For this review, take the finished solid that the model builds, in its own axes (mm). Face numbers are marked on the shaded views. A direction names the side the tool comes from. Round coordinates to 2 decimals unless told otherwise and drop trailing zeros. Write each loop counter-clockwise with the first axis right and the second up, starting at its lowest first coordinate (ties: lowest second). Pieces come first, ordered by that corner, then holes. Notation, with made-up numbers: (9, -8.5) -> (58, -8.5) arc R24 cw to (58, 13.5) -> close; hole circle Ø4 at (-13, 9.25). An arc over 180 degrees is marked (long way). Answer as CSV lines item,"result". Start each with the question number.
Item 1: Mouldability with a two-part tool opening along Y and no side actions: class the marked faces 4, 5 and 6 as +Y half, -Y half, draft (parallel to the pull), parting line (faces both ways), or undercut.
Item 2: Machinability: for the marked faces 1, 2 and 3, which of the approach directions +Z, -Z, +X, -X, +Y, -Y give a long, thin tool a straight path to every point of the face, cutting with its end or side? Answer none if there is none.
Item 3: Wall thickness on probe 1 along Y at (x, z) = (-0.25, 2.5); probe 2 along Y at (x, z) = (-4, 9.75): over which ranges is each line inside the solid? List them lowest first. Write a range as from..to.
Item 4: Take a section at C-C on y = 0.25. Give the boundary of the cut face in (x, z).
Item 5: Take a section at D-D on x = -1.75. Give the boundary of the cut face in (y, z), then the cut area to 3 significant figures.
Item 6: Take a section at B-B on z = 8.5. Count the separate pieces of the cut face and the enclosed holes in it, then the cut area to 3 significant figures.
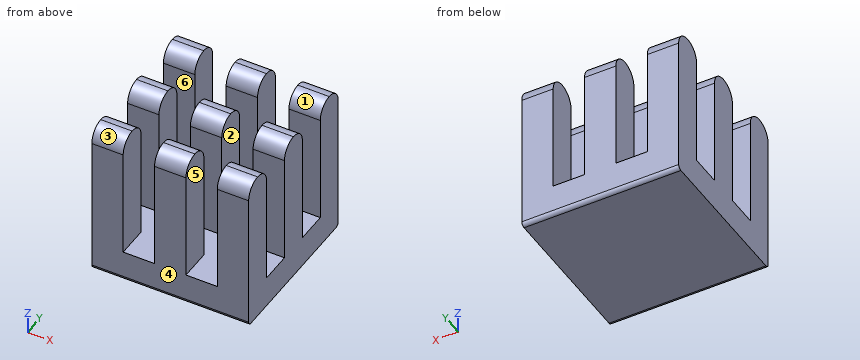
```python
from build123d import *

# Parameters (mm, degrees)
BOX_W                  = 10
BOX_H                  = 10
BOX_DEPTH              = 10
SKETCH_W               = 2
SKETCH_H               = 10
POCKET_DEPTH           = 10.001
LINEARPATTERN_COUNT    = 2
LINEARPATTERN_PITCH    = 4
SKETCH001_W            = 2
SKETCH001_H            = 10
POCKET001_DEPTH        = 10.001
LINEARPATTERN001_COUNT = 2
LINEARPATTERN001_PITCH = 4
FILLET_R               = 0.999
FILLET001_R            = 0.25


with BuildPart() as part:
    # Box → Box (new body)
    with BuildSketch(Plane(origin=(-5, -5, 0), x_dir=(1, 0, 0), z_dir=(0, 0, 1))):
        with Locations((5, 5)):
            Rectangle(BOX_W, BOX_H)
    extrude(amount=BOX_DEPTH)

    # Sketch → Pocket (cut, through all)
    with BuildSketch(Plane(origin=(-5, -5, 0), x_dir=(1, 0, 0), z_dir=(0, -1, 0))):
        with Locations((3, 7)):
            Rectangle(SKETCH_W, SKETCH_H)
    pocket = extrude(amount=-POCKET_DEPTH, mode=Mode.SUBTRACT)

    # LinearPattern: Pocket ×2
    with Locations(*[(i * LINEARPATTERN_PITCH, 0, 0) for i in range(1, LINEARPATTERN_COUNT)]):
        add(pocket, mode=Mode.SUBTRACT)

    # Sketch001 → Pocket001 (cut, through all)
    with BuildSketch(Plane(origin=(5, -5, 0), x_dir=(0, 1, 0), z_dir=(1, 0, 0))):
        with Locations((3, 7)):
            Rectangle(SKETCH001_W, SKETCH001_H)
    pocket001 = extrude(amount=-POCKET001_DEPTH, mode=Mode.SUBTRACT)

    # LinearPattern001: Pocket001 ×2
    with Locations(*[(0, i * LINEARPATTERN001_PITCH, 0) for i in range(1, LINEARPATTERN001_COUNT)]):
        add(pocket001, mode=Mode.SUBTRACT)

    # Fillet
    fillet_edges = [part.edges().sort_by_distance(p)[0] for p in [
        (-4, -5, 10),
        (-4, -3, 10),
        (0, -5, 10),
        (0, -3, 10),
        (4, -5, 10),
        (4, -3, 10),
        (4, -1, 10),
        (4, 1, 10),
        (0, 1, 10),
        (0, -1, 10),
        (-4, -1, 10),
        (-4, 1, 10),
        (-4, 3, 10),
        (-4, 5, 10),
        (0, 5, 10),
        (0, 3, 10),
        (4, 5, 10),
        (4, 3, 10),
    ]]
    fillet(fillet_edges, radius=FILLET_R)

    # Fillet001
    fillet001_edges = [part.edges().sort_by_distance(p)[0] for p in [
        (0, -5, 0),
        (0, 5, 0),
    ]]
    fillet(fillet001_edges, radius=FILLET001_R)


solid = part.part
```
Output values:
1,face 4,"-Y half"
1,face 5,"draft"
1,face 6,"undercut"
2,face 1,"+Z, +X, -X"
2,face 2,"+Z, +Y, -Y"
2,face 3,"+Z, +X, -X, -Y"
3,probe 1,"y = -5..-3, -1..1, 3..5"
3,probe 2,"y = -4.66..-3.34, -0.66..0.66, 3.34..4.66"
4,outline,"(-5, 0) -> (5, 0) -> (5, 9.97) -> (3, 9.97) -> (3, 2) -> (1, 2) -> (1, 9.97) -> (-1, 9.97) -> (-1, 2) -> (-3, 2) -> (-3, 9.97) -> (-5, 9.97) -> close"
5,outline,"(-5, 0.25) arc R0.25 ccw to (-4.75, 0) -> (4.75, 0) arc R0.25 ccw to (5, 0.25) -> (5, 2) -> (-5, 2) -> close"
5,area,"20.0 mm^2"
6,separate pieces,"9"
6,enclosed holes,"0"
6,area,"36.0 mm^2"
